```python
from build123d import *

# Parameters (mm, degrees)
BOSS_EXTRUDE1_DEPTH     = 2.5
SKETCH3_W               = 3
SKETCH3_H               = 19
BOSS_EXTRUDE2_DEPTH     = 35
LPATTERN1_COUNT         = 2
LPATTERN1_PITCH         = 35
CUT_EXTRUDE2_DEPTH      = 54.866960969
CUT_EXTRUDE2_DEPTH_BACK = 10
SKETCH6_R               = 1.6
SKETCH8_R               = 1.6
CUT_EXTRUDE4_DEPTH      = 56.523864095
FILLET1_R               = 2
FILLET2_R               = 2


with BuildPart() as part:
    # Sketch2 → Boss-Extrude1 (new body)
    with BuildSketch(Plane.XY):
        with BuildLine():
            Line((-32, -7.690598923), (-32, 7.690598923))
            ThreePointArc((-32, 7.690598923), (-31.464101615, 9.690598923), (-30, 11.154700538))
            Line((-30, 11.154700538), (-6, 25.011106999))
            ThreePointArc((-6, 25.011106999), (-2, 25.011106999), (0, 21.547005384))
            Line((0, 21.547005384), (0, -21.547005384))
            ThreePointArc((0, -21.547005384), (-2, -25.011106999), (-6, -25.011106999))
            Line((-6, -25.011106999), (-30, -11.154700538))
            ThreePointArc((-30, -11.154700538), (-31.464101615, -9.690598923), (-32, -7.690598923))
        make_face()
    boss_extrude1 = extrude(amount=BOSS_EXTRUDE1_DEPTH)

    # Sketch3 → Boss-Extrude2 (add)
    with BuildSketch(Plane.XY.offset(2.5)):
        with Locations((-1.5, 0)):
            Rectangle(SKETCH3_W, SKETCH3_H)
    extrude(amount=BOSS_EXTRUDE2_DEPTH)

    # LPattern1: Boss-Extrude1 ×2
    with Locations(*[(0, 0, i * LPATTERN1_PITCH) for i in range(1, LPATTERN1_COUNT)]):
        add(boss_extrude1)

    # Sketch6 → Cut-Extrude2 (cut, two sides: drawn at the far end of the back side and taken through both)
    with BuildSketch(Plane.XY.offset(2.5).offset(-CUT_EXTRUDE2_DEPTH_BACK)):
        with Locations(Location((-26, 8, 0), (0, 0, 180))):
            Circle(SKETCH6_R)
        with Locations(Location((-26, -8, 0), (0, 0, 180))):
            Circle(SKETCH6_R)
    extrude(amount=CUT_EXTRUDE2_DEPTH + CUT_EXTRUDE2_DEPTH_BACK, mode=Mode.SUBTRACT)

    # Sketch8 → Cut-Extrude4 (cut, through all)
    with BuildSketch(Plane.XY.offset(37.5)):
        with Locations((-5, 16.511106999)):
            Circle(SKETCH8_R)
        with Locations((-5, -14.011106999)):
            Circle(SKETCH8_R)
    extrude(amount=-CUT_EXTRUDE4_DEPTH, mode=Mode.SUBTRACT)

    # Fillet1
    fillet1_edges = [part.edges().sort_by_distance(p)[0] for p in [
        (-1.5, 9.5, 2.5),
        (-1.5, -9.5, 2.5),
        (-1.5, -9.5, 35),
        (-1.5, 9.5, 35),
    ]]
    fillet(fillet1_edges, radius=FILLET1_R)

    # Fillet2
    fillet2_edges = [part.edges().sort_by_distance(p)[0] for p in [
        (-3, 0, 2.5),
        (-3, 0, 35),
    ]]
    fillet(fillet2_edges, radius=FILLET2_R)


solid = part.part
```
Work out the finished part from the listing and answer in its coordinate system (mm). A direction names the side the tool comes from. Give positions to 0.01 mm unless a question says otherwise; leave off trailing zeros. Order: outer loops, then holes, each group sorted by start corner. A loop starts at its lowest first (then second) coordinate and runs counter-clockwise, first axis right, second up. Notation, with made-up numbers: (25.5, -3.5) - (56.5, -3.5) arc R5 ccw to (56.5, 3.5) - close; hole circle Ø8 at (-27, 18.25). An arc over 180 degrees is marked (long way). One line per item, written item: value. Start each with the question number.
1. Each of these flat-tipped pins is pushed along its axis until it touches: pin 1 Ø12 at (y, z) = (5, 14) entering from -X; pin 2 Ø1.9 at (x, y) = (-5, -14.01) entering from +Z; pin 3 Ø15 at (y, z) = (-3.5, 26) entering from -X; pin 4 Ø10 at (x, z) = (-5.5, 29.5) entering from -Y. Where does it stop, or does it pass through?
2. Which of the six approach directions +Z, -Z, +X, -X, +Y, -Y give full straight-line access (tool end or side, diameter ignored) to faces 1 (the face through (-2, 9.5, 19)), 2 (the face through (-3.6, -0.16, 34.43)), 3 (the face through (-32, 0, 1))?
3. Consider line 1 (Z direction, x = -11, y = 18.5); line 2 (Y direction, x = -26, z = 36.7); line 3 (Y direction, x = -5, z = 1.6). Determine where each line is inside the solid, lowest interval first.
4. Section C-C, the plane x = -22.5 is taken. Write down the section's boundary in (y, z).
5. For a pull along Z with two mould halves and no side action, classify faces 4 (the face through (-2.05, 25.04, 1.23)), 5 (the face through (-1.98, -10.1, 34.43)), 6 (the face through (-3.6, -0.16, 3.07)) as released by +Z, released by -Z, zero draft, split by the parting line, or undercut.
6. Section D-D, the plane z = 12 is taken. Write down the section's boundary in (x, y), then the cut area to 3 significant figures.
7. Section A-A, the plane x = -26 is taken. Write down the section's boundary in (y, z).
8. Section B-B, the plane y = -2 is taken. Write down the section's boundary in (x, z), then the cut area to 3 significant figures.
Filled sheet:
1. pin 1: x = -3
1. pin 2: through
1. pin 3: x = -3.06
1. pin 4: y = -9.75
2. face 1: +X, -X, +Y
2. face 2: -X, +Y, -Y
2. face 3: +Z, -Z, -X, +Y, -Y
3. line 1: 0 to 2.5, 35 to 37.5
3. line 2: -13.46 to -9.6, -6.4 to 6.4, 9.6 to 13.46
3. line 3: -25.42 to -15.61, -12.41 to 14.91, 18.11 to 25.42
4. outline: (-15.48, 0) - (15.48, 0) - (15.48, 2.5) - (-15.48, 2.5) - close; (-15.48, 35) - (15.48, 35) - (15.48, 37.5) - (-15.48, 37.5) - close
5. face 4: zero draft
5. face 5: undercut
5. face 6: undercut
6. outline: (-3, -9.5) - (0, -9.5) - (0, 9.5) - (-3, 9.5) - close
6. area: 57.0 mm²
7. outline: (-13.46, 0) - (-9.6, 0) - (-9.6, 2.5) - (-13.46, 2.5) - close; (-13.46, 35) - (-9.6, 35) - (-9.6, 37.5) - (-13.46, 37.5) - close; (-6.4, 0) - (6.4, 0) - (6.4, 2.5) - (-6.4, 2.5) - close; (-6.4, 35) - (6.4, 35) - (6.4, 37.5) - (-6.4, 37.5) - close; (9.6, 0) - (13.46, 0) - (13.46, 2.5) - (9.6, 2.5) - close; (9.6, 35) - (13.46, 35) - (13.46, 37.5) - (9.6, 37.5) - close
8. outline: (-32, 0) - (0, 0) - (0, 37.5) - (-32, 37.5) - (-32, 35) - (-5, 35) arc R2 cw to (-3, 33) - (-3, 4.5) arc R2 cw to (-5, 2.5) - (-32, 2.5) - close
8. area: 259 mm²
